CAD build for the part. Positions are in the model's coordinates, mm. Face numbers are marked on the shaded views. Coordinates: 2 decimals unless noted, no trailing zeros. Loops run counter-clockwise (first coordinate to the right, second up) from the corner with the lowest first, then second, coordinate; pieces in that order, holes last. Notation, with made-up numbers: (68.5, 65.25) -> (114.5, 65.25) arc R13 cw to (114.5, 86.25) -> close; hole circle Ø3 at (20.25, 30). An arc over 180 degrees is marked (long way). Return JSON: item names as keys, results as strings. Group by question number.
(1) Saw through at B-B on x = 2.5. Write the cut outline in (y, z), then the cut area to 3 significant figures.
(2) Mould opens along Z. For the marked faces 1, 2 and 3 say: pulls with the +Z half, pulls with the -Z half, needs draft (parallel to the pull), parting line crosses it, or undercut.
(3) Flat gauge pin, fed straight in: pin 1 Ø2 at (x, z) = (2.5, 0) entering from +Y. Where does the tip first touch, or does it go through?
(4) Saw through at A-A on z = 0. Write the cut outline in (x, y), then the cut area to 3 significant figures.
(5) Saw through at C-C on y = 10.25. Write the cut outline in (x, z), then the cut area to 3 significant figures.
(6) Saw through at D-D on z = -1.5. Write the cut outline in (x, y).
(7) Probe L1, parallel to X at y = 3.25, z = 0; L2, parallel to Z at x = -4, y = 10.5; L3, parallel to X at y = 3.25, z = -1.5. List the from-to ranges inside material, lowest first.
```python
from build123d import *

# Parameters (mm, degrees)
SKETCH_1_W          = 14
SKETCH_1_H          = 9
EXTRUDE_1_DEPTH     = 14
FILLET_1_R          = 1
CUT_EXTRUDE_2_REACH = 18.286
SKETCH_3_R          = 1.75


with BuildPart() as part:
    # 草图1 → 凸台-拉伸1 (new body)
    with BuildSketch(Plane(origin=(0, 0, 0), x_dir=(1, 0, 0), z_dir=(0, 1, 0))):
        Rectangle(SKETCH_1_W, SKETCH_1_H)
    extrude(amount=EXTRUDE_1_DEPTH)

    # 圆角1
    fillet_1_edges = [part.edges().sort_by_distance(p)[0] for p in [
        (7, 7, 4.5),
        (-7, 7, 4.5),
        (-7, 7, -4.5),
        (7, 7, -4.5),
    ]]
    fillet(fillet_1_edges, radius=FILLET_1_R)

    # 草图3 → 切除-拉伸2 (cut, up to next)
    with BuildSketch(Plane(origin=(0, 14, 0), x_dir=(1, 0, 0), z_dir=(0, 1, 0)), mode=Mode.PRIVATE) as cut_extrude_2_sk1:
        with Locations(Location((-2.5, 0, 0), (0, 0, 270))):
            Circle(SKETCH_3_R)
    cut_extrude_2_tool1 = extrude(cut_extrude_2_sk1.sketch, amount=-CUT_EXTRUDE_2_REACH, mode=Mode.PRIVATE) & part.part
    # 草图3 → 切除-拉伸2 (cut, up to next)
    with BuildSketch(Plane(origin=(0, 14, 0), x_dir=(1, 0, 0), z_dir=(0, 1, 0)), mode=Mode.PRIVATE) as cut_extrude_2_sk2:
        with Locations(Location((2.5, 0, 0), (0, 0, 270))):
            Circle(SKETCH_3_R)
    cut_extrude_2_tool2 = extrude(cut_extrude_2_sk2.sketch, amount=-CUT_EXTRUDE_2_REACH, mode=Mode.PRIVATE) & part.part
    add(cut_extrude_2_tool1.solids().sort_by_distance((-2.5, 14, 0))[0], mode=Mode.SUBTRACT)
    add(cut_extrude_2_tool2.solids().sort_by_distance((2.5, 14, 0))[0], mode=Mode.SUBTRACT)


solid = part.part
```
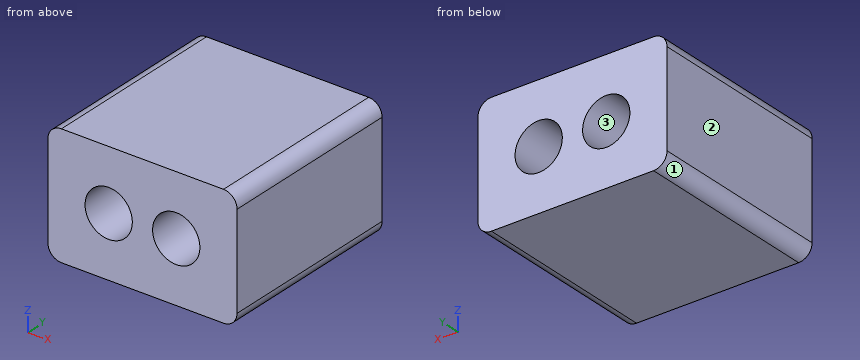
Geometry results:
{
 "1": {"outline": "(0, -4.5) -> (14, -4.5) -> (14, -1.75) -> (0, -1.75) -> close; (0, 1.75) -> (14, 1.75) -> (14, 4.5) -> (0, 4.5) -> close", "area": "77.0 mm²"},
 "2": {"face 1": "pulls with the -Z half", "face 2": "needs draft", "face 3": "undercut"},
 "3": {"pin 1": "through"},
 "4": {"outline": "(-7, 0) -> (-4.25, 0) -> (-4.25, 14) -> (-7, 14) -> close; (-0.75, 0) -> (0.75, 0) -> (0.75, 14) -> (-0.75, 14) -> close; (4.25, 0) -> (7, 0) -> (7, 14) -> (4.25, 14) -> close", "area": "98.0 mm²"},
 "5": {"outline": "(-7, -3.5) arc R1 ccw to (-6, -4.5) -> (6, -4.5) arc R1 ccw to (7, -3.5) -> (7, 3.5) arc R1 ccw to (6, 4.5) -> (-6, 4.5) arc R1 ccw to (-7, 3.5) -> close; hole circle Ø3.5 at (-2.5, 0); hole circle Ø3.5 at (2.5, 0)", "area": "106 mm²"},
 "6": {"outline": "(-7, 0) -> (-3.4, 0) -> (-3.4, 14) -> (-7, 14) -> close; (-1.6, 0) -> (1.6, 0) -> (1.6, 14) -> (-1.6, 14) -> close; (3.4, 0) -> (7, 0) -> (7, 14) -> (3.4, 14) -> close"},
 "7": {"L1": "-7 to -4.25, -0.75 to 0.75, 4.25 to 7", "L2": "-4.5 to -0.9, 0.9 to 4.5", "L3": "-7 to -3.4, -1.6 to 1.6, 3.4 to 7"}
}
